CAD build for the part. Positions are in the model's coordinates, mm. A direction names the side the tool comes from. Give positions to 0.01 mm unless a question says otherwise; leave off trailing zeros. Order: outer loops, then holes, each group sorted by start corner. A loop starts at its lowest first (then second) coordinate and runs counter-clockwise, first axis right, second up. Notation, with made-up numbers: M 17.25,1.25 L 56.25,1.25 A33 cw 56.25,39.25 Z; hole C -35,37.5 d3. An arc over 180 degrees is marked long. Put each result on its own line as item: value. Start each with the question number.
1) Tool access for faces 4 (the face through (0, 15, -4)), 5 (the face through (-6.324, 6.338, -4.032)): list every direction of +Z, -Z, +X, -X, +Y, -Y with a clear straight run to the whole face (end or side of a thin tool).
2) Cut at A-A (x = 5.5). Write the cut outline in (y, z).
3) Drill centre lines: line 1 (X direction, y = 9.4, z = 0); line 2 (X direction, y = 14, z = 0) (3 decimals); line 3 (Y direction, x = -8.25, z = 4.5). Where is each one in solid material? Low to high. Write a range as [from, to].
4) Cut at D-D (x = 7.75). Write the cut outline in (y, z), and give its area (3 significant figures).
5) Cut at C-C (x = -7). Write the cut outline in (y, z), and give its area (3 significant figures).
6) Pin check, flat tips, straight feed: pin 1 (1 mm diameter, centred on x = 2, y = 11, fed in from -Z); pin 2 (1 mm diameter, centred on y = 11, z = -4.5, fed in from +X); pin 3 (4 mm diameter, centred on x = -7.5, y = 5, fed in from +Z); pin 4 (4 mm diameter, centred on x = 0, z = 0, fed in from +Y). Stop position of each tip, or through.
7) Two-plate mould, pull along X, no slides. Class faces 1 (the face through (5, 0, 0)), 2 (the face through (9.3, 13.77, 2.06)), 3 (the face through (0, 10, 5)): released by +X, released by -X, zero draft, split by the parting line, or undercut.
8) Cut at B-B (y = 9.25). Write the cut outline in (x, z).
```python
from build123d import *


with BuildPart() as part:
    # Sketch1 → Revolve1 (revolve)
    with BuildSketch(Plane.XY, mode=Mode.PRIVATE) as revolve1_sk:
        Polygon((7.5, 0), (7.5, 12.5), (9.525, 12.5), (9.525, 15), (3.3, 15), (3.3, 11), (5, 11), (5, 9), (4.3235, 9), (5, 8.5), (4.3235, 8), (5, 7.5), (4.3235, 7), (5, 6.5), (4.3235, 6), (5, 5.5), (4.3235, 5), (5, 4.5), (4.3235, 4), (5, 3.5), (4.3235, 3), (5, 2.5), (4.3235, 2), (5, 1.5), (4.3235, 1), (5, 0.5), (4.3235, 0), align=None)
    revolve(revolve1_sk.sketch.rotate(Axis((0, 0, 0), (0, 1, 0)), 90), axis=Axis((0, 0, 0), (0, 1, 0)))  # turned: the seam where the file's is


solid = part.part
```
Solution:
1. face 4: +Z, -Z, +X, -X, +Y
1. face 5: -Y
2. outline: M 0,-5.1 L 12.5,-5.1 L 12.5,-7.78 L 15,-7.78 L 15,7.78 L 12.5,7.78 L 12.5,5.1 L 0,5.1 Z
3. line 1: [-7.5, -5], [5, 7.5]
3. line 2: [-9.525, -3.3], [3.3, 9.525]
3. line 3: [12.5, 15]
4. outline: M 12.5,-5.54 L 15,-5.54 L 15,5.54 L 12.5,5.54 Z
4. area: 27.7 mm²
5. outline: M 0,-2.69 L 12.5,-2.69 L 12.5,-6.46 L 15,-6.46 L 15,6.46 L 12.5,6.46 L 12.5,2.69 L 0,2.69 Z
5. area: 99.6 mm²
6. pin 1: z = -7.35
6. pin 2: x = 6.34
6. pin 3: z = 5.1
6. pin 4: through
7. face 1: zero draft
7. face 2: split by the parting line
7. face 3: undercut
8. outline: C 0,0 d15; hole C 0,0 d10
